```python
from build123d import *

# Parameters (mm, degrees)
F0_W      = 508
F0_H      = 254
F1_DEPTH  = 2.54
F2_W      = 2.54
F2_H      = 254
F3_DEPTH  = 203.2
F4_W      = 505.46
F4_H      = 2.54
F5_DEPTH  = 203.2
F6_W      = 2.54
F6_H      = 251.46
F7_DEPTH  = 203.2
F8_W      = 502.92
F8_H      = 2.54
F9_DEPTH  = 203.2
F10_W     = 50.8
F10_H     = 88.9
F11_DEPTH = 25.4
F12_W     = 50.8
F12_H     = 25.4
F13_DEPTH = 25.4


with BuildPart() as f1:
    # F0 (on Top) → F1 (new body)
    with BuildSketch(Plane.XY):
        Rectangle(F0_W, F0_H)
    extrude(amount=F1_DEPTH)

    # F2 (on face) → F3 (join)
    with BuildSketch(Plane.XY.offset(2.54)):
        with Locations((-252.73, 0)):
            Rectangle(F2_W, F2_H)
    extrude(amount=F3_DEPTH)

    # F4 (on face) → F5 (join)
    with BuildSketch(Plane.XY.offset(2.54)):
        with Locations((1.27, 125.73)):
            Rectangle(F4_W, F4_H)
    extrude(amount=F5_DEPTH)

    # F6 (on face) → F7 (join)
    with BuildSketch(Plane.XY.offset(2.54)):
        with Locations((252.73, -1.27)):
            Rectangle(F6_W, F6_H)
    extrude(amount=F7_DEPTH)

    # F8 (on face) → F9 (join)
    with BuildSketch(Plane.XY.offset(2.54)):
        with Locations((0, -125.73)):
            Rectangle(F8_W, F8_H)
    extrude(amount=F9_DEPTH)

    # F10 (on face) → F11 (cut)
    with BuildSketch(Plane.YZ.offset(-251.46)):
        with Locations((8.812193, 46.99)):
            Rectangle(F10_W, F10_H)
    extrude(amount=-F11_DEPTH, mode=Mode.SUBTRACT)

    # F12 (on face) → F13 (cut)
    with BuildSketch(Plane(origin=(-254, 0, 0), x_dir=(0, -1, 0), z_dir=(-1, 0, 0))):
        with Locations((71.237722, 77.256631)):
            Rectangle(F12_W, F12_H)
    extrude(amount=-F13_DEPTH, mode=Mode.SUBTRACT)


solid = f1.part
```
CAD build for the part. Positions are in the model's coordinates, mm. A direction names the side the tool comes from. Coordinates: 2 decimals unless noted, no trailing zeros. Write each loop counter-clockwise with the first axis right and the second up, starting at its lowest first coordinate (ties: lowest second). Pieces come first, ordered by that corner, then holes. Notation, with made-up numbers: (74.5, 89) -> (96.5, 89) arc R26 cw to (96.5, 110) -> close; hole circle Ø9 at (51, 87). An arc over 180 degrees is marked (long way). Return JSON: item names as keys, results as strings. Group by question number.
Q1. Cut at B-B, the plane z = 158. Give the cut face in (x, y).
Q2. Flat gauge pin, fed straight in: pin 1 (0.8 mm diameter, centred on x = -253, y = 16.5, fed in from -Z). Where does the tip first touch, or does it go through?
Q3. Drill centre lines: line 1 (X direction, y = -90, z = 114.5); line 2 (Y direction, x = -124, z = 188); line 3 (Z direction, x = -74, y = 49.5). Where is each one in solid material? Low to high.
Q4. Cut at A-A, the plane y = -70.5. Give the cut face in (x, z).
Q5. Cut at C-C, the plane y = -30. Give the cut face in (x, z).
Q6. Which spindle directions (+Z, -Z, +X, -X, +Y, -Y) get a long thin tool onto all of the face, cutting with end or side? Do faces 1 (the face through (-4, 2, 0)), 2 (the face through (-4, -124.46, 103)). Say none if no direction does.
Q7. Pull direction X, two halves, no side cores. Call faces 3 (the face through (-254, -2, 101)), 4 (the face through (2, -2, 2.54)), 5 (the face through (-4, 127, 101)): released by +X, released by -X, zero draft, split by the parting line, or undercut.
Q8. Cut at D-D, the plane z = 57.5. Give the cut face in (x, y), then the cut area to 3 significant figures.
Returned:
{
 "1": {"outline": "(-254, -127) -> (254, -127) -> (254, 127) -> (-254, 127) -> close; hole (-251.46, -124.46) -> (251.46, -124.46) -> (251.46, 124.46) -> (-251.46, 124.46) -> close"},
 "2": {"pin 1": "stops at z = 0"},
 "3": {"line 1": "x = -254 to -251.46, 251.46 to 254", "line 2": "y = -127 to -124.46, 124.46 to 127", "line 3": "z = 0 to 2.54"},
 "4": {"outline": "(-254, 0) -> (254, 0) -> (254, 205.74) -> (251.46, 205.74) -> (251.46, 2.54) -> (-251.46, 2.54) -> (-251.46, 64.56) -> (-254, 64.56) -> close; (-254, 89.96) -> (-251.46, 89.96) -> (-251.46, 205.74) -> (-254, 205.74) -> close"},
 "5": {"outline": "(-254, 0) -> (254, 0) -> (254, 205.74) -> (251.46, 205.74) -> (251.46, 2.54) -> (-251.46, 2.54) -> (-251.46, 205.74) -> (-254, 205.74) -> close"},
 "6": {"face 1": "-Z, +X, -X, +Y, -Y", "face 2": "+Z"},
 "7": {"face 3": "released by -X", "face 4": "undercut", "face 5": "zero draft"},
 "8": {"outline": "(-254, -127) -> (254, -127) -> (254, 127) -> (-254, 127) -> (-254, 34.21) -> (-251.46, 34.21) -> (-251.46, 124.46) -> (251.46, 124.46) -> (251.46, -124.46) -> (-251.46, -124.46) -> (-251.46, -16.59) -> (-254, -16.59) -> close", "area": "3,720 mm2"}
}
